Design review of the part built by this model. Coordinates are the model's own, in mm. A direction names the side the tool comes from. Coordinates: 2 decimals unless noted, no trailing zeros. Write item = value, one per line.
```python
from build123d import *

# Parameters (mm, degrees)
SKETCH_1_R          = 13
SKETCH_1_R_2        = 1.65
EXTRUDE_1_DEPTH     = 5
SKETCH_2_R          = 2
CUT_EXTRUDE_2_DEPTH = 5
CUT_EXTRUDE_START   = -5
CUT_EXTRUDE_3_DEPTH = 5
FILLET_1_R          = 2
FILLET_2_R          = 2
FILLET_3_R          = 2
CUT_EXTRUDE_5_DEPTH = 5
SKETCH_9_R          = 2
CUT_EXTRUDE_6_DEPTH = 10
SKETCH_10_R         = 2
CUT_EXTRUDE_7_DEPTH = 10
SKETCH_11_W         = 30
SKETCH_11_H         = 5
EXTRUDE_2_DEPTH     = 5
SKETCH_12_W         = 28.554441288
SKETCH_12_H         = 5
EXTRUDE_3_DEPTH     = 5


with BuildPart() as part:
    # 草图1 → 凸台-拉伸1 (new body)
    with BuildSketch(Plane.XY):
        with BuildLine():
            Line((0, 25), (450, 25))
            ThreePointArc((450, 25), (475, 0), (450, -25))
            Line((450, -25), (0, -25))
            ThreePointArc((0, -25), (-25, 0), (0, 25))
        make_face()
        Circle(SKETCH_1_R, mode=Mode.SUBTRACT)
        with Locations((17.5, 0)):
            Circle(SKETCH_1_R_2, mode=Mode.SUBTRACT)
        with Locations((0, -17.5)):
            Circle(SKETCH_1_R_2, mode=Mode.SUBTRACT)
        with Locations((-17.5, 0)):
            Circle(SKETCH_1_R_2, mode=Mode.SUBTRACT)
        with Locations((0, 17.5)):
            Circle(SKETCH_1_R_2, mode=Mode.SUBTRACT)
        with Locations((450, 0)):
            Circle(SKETCH_1_R, mode=Mode.SUBTRACT)
        with Locations((432.5, 0)):
            Circle(SKETCH_1_R_2, mode=Mode.SUBTRACT)
        with Locations((450, 17.5)):
            Circle(SKETCH_1_R_2, mode=Mode.SUBTRACT)
        with Locations((450, -17.5)):
            Circle(SKETCH_1_R_2, mode=Mode.SUBTRACT)
        with Locations((467.5, 0)):
            Circle(SKETCH_1_R_2, mode=Mode.SUBTRACT)
    extrude(amount=EXTRUDE_1_DEPTH)

    # 草图2 → 切除-拉伸2 (cut)
    with BuildSketch(Plane.XY.offset(5)):
        with Locations((290, 12.5)):
            Circle(SKETCH_2_R)
        with Locations((290, 0)):
            Circle(SKETCH_2_R)
        with Locations((290, -12.5)):
            Circle(SKETCH_2_R)
        with Locations((160, 12.5)):
            Circle(SKETCH_2_R)
        with Locations((160, 0)):
            Circle(SKETCH_2_R)
        with Locations((160, -12.5)):
            Circle(SKETCH_2_R)
    extrude(amount=-CUT_EXTRUDE_2_DEPTH, mode=Mode.SUBTRACT)

    # 草图4 → 切除-拉伸3 (cut)
    with BuildSketch(Plane.XY.offset(5).offset(CUT_EXTRUDE_START)):
        with BuildLine():
            Line((74.250402222, 0), (22.107690969, -17.5))
            ThreePointArc((22.107690969, -17.5), (20.333388811, -16.422958207), (20.470084231, -14.351851852))
            ThreePointArc((20.470084231, -14.351851852), (25, 0), (20.470084231, 14.351851852))
            ThreePointArc((20.470084231, 14.351851852), (20.333388811, 16.422958207), (22.107690969, 17.5))
            Line((22.107690969, 17.5), (74.250402222, 0))
        make_face()
        Polygon((82.107690969, -2.637042643), (126.393113474, -17.5), (37.822268465, -17.5), align=None)
        Polygon((37.822268465, 17.5), (126.393113474, 17.5), (82.107690969, 2.637042643), align=None)
        Polygon((142.107690969, 17.5), (142.107690969, -17.5), (89.964979717, 0), align=None)
    cut_extrude_3 = extrude(amount=CUT_EXTRUDE_3_DEPTH, mode=Mode.SUBTRACT)

    # 圆角1
    fillet_1_edges = [part.edges().sort_by_distance(p)[0] for p in [
        (142.107690969, 17.5, 2.5),
    ]]
    fillet(fillet_1_edges, radius=FILLET_1_R)

    # 圆角2
    fillet_2_edges = [part.edges().sort_by_distance(p)[0] for p in [
        (37.822268465, -17.5, 2.5),
        (82.107690969, -2.637042643, 2.5),
        (126.393113474, -17.5, 2.5),
        (89.964979717, 0, 2.5),
        (142.107690969, -17.5, 2.5),
        (126.393113474, 17.5, 2.5),
        (82.107690969, 2.637042643, 2.5),
        (37.822268465, 17.5, 2.5),
        (74.250402222, 0, 2.5),
    ]]
    fillet(fillet_2_edges, radius=FILLET_2_R)

    # 镜向1: 切除-拉伸3 across plane
    add(cut_extrude_3.mirror(Plane(origin=(225, 0, 0), x_dir=(0, 0, 1), z_dir=(1, 0, 0))), mode=Mode.SUBTRACT)

    # 圆角3
    fillet_3_edges = [part.edges().sort_by_distance(p)[0] for p in [
        (375.749597778, 0, 2.5),
        (367.892309031, -2.637042643, 2.5),
        (412.177731535, -17.5, 2.5),
        (323.606886526, -17.5, 2.5),
        (307.892309031, 17.5, 2.5),
        (360.035020283, 0, 2.5),
        (307.892309031, -17.5, 2.5),
        (367.892309031, 2.637042643, 2.5),
        (323.606886526, 17.5, 2.5),
        (412.177731535, 17.5, 2.5),
    ]]
    fillet(fillet_3_edges, radius=FILLET_3_R)

    # 草图8 → 切除-拉伸5 (cut)
    with BuildSketch(Plane.XY.offset(5)):
        with BuildLine():
            Line((198.641718603, 17.5), (251.358281397, 17.5))
            ThreePointArc((251.358281397, 17.5), (253.321552393, 15.881532429), (252.107332949, 13.645566994))
            Line((252.107332949, 13.645566994), (225.749051552, 2.998802443))
            ThreePointArc((225.749051552, 2.998802443), (225, 2.853235449), (224.250948448, 2.998802443))
            Line((224.250948448, 2.998802443), (197.892667051, 13.645566994))
            ThreePointArc((197.892667051, 13.645566994), (196.678447607, 15.881532429), (198.641718603, 17.5))
        make_face()
        with BuildLine():
            Line((175, 14.535156791), (175, -14.535156791))
            ThreePointArc((175, -14.535156791), (175.881541933, -16.193183193), (177.749051552, -16.389589796))
            Line((177.749051552, -16.389589796), (213.733857169, -1.854433006))
            ThreePointArc((213.733857169, -1.854433006), (214.984805617, 0), (213.733857169, 1.854433006))
            Line((213.733857169, 1.854433006), (177.749051552, 16.389589796))
            ThreePointArc((177.749051552, 16.389589796), (175.881541933, 16.193183193), (175, 14.535156791))
        make_face()
        with BuildLine():
            Line((198.641718603, -17.5), (251.358281397, -17.5))
            ThreePointArc((251.358281397, -17.5), (253.321552393, -15.881532429), (252.107332949, -13.645566994))
            Line((252.107332949, -13.645566994), (225.749051552, -2.998802443))
            ThreePointArc((225.749051552, -2.998802443), (225, -2.853235449), (224.250948448, -2.998802443))
            Line((224.250948448, -2.998802443), (197.892667051, -13.645566994))
            ThreePointArc((197.892667051, -13.645566994), (196.678447607, -15.881532429), (198.641718603, -17.5))
        make_face()
        with BuildLine():
            Line((275, 14.535156791), (275, -14.535156791))
            ThreePointArc((275, -14.535156791), (274.118458067, -16.193183193), (272.250948448, -16.389589796))
            Line((272.250948448, -16.389589796), (236.266142831, -1.854433006))
            ThreePointArc((236.266142831, -1.854433006), (235.015194383, 0), (236.266142831, 1.854433006))
            Line((236.266142831, 1.854433006), (272.250948448, 16.389589796))
            ThreePointArc((272.250948448, 16.389589796), (274.118458067, 16.193183193), (275, 14.535156791))
        make_face()
    extrude(amount=-CUT_EXTRUDE_5_DEPTH, mode=Mode.SUBTRACT)

    # 草图9 → 切除-拉伸6 (cut)
    with BuildSketch(Plane.XY.offset(5)):
        with Locations((38, 19)):
            Circle(SKETCH_9_R)
        with Locations((38, -19)):
            Circle(SKETCH_9_R)
    cut_extrude_6 = extrude(amount=-CUT_EXTRUDE_6_DEPTH, mode=Mode.SUBTRACT)

    # 镜向2: 切除-拉伸6 across plane
    add(cut_extrude_6.mirror(Plane(origin=(225, 0, 0), x_dir=(0, 0, 1), z_dir=(1, 0, 0))), mode=Mode.SUBTRACT)

    # 草图10 → 切除-拉伸7 (cut)
    with BuildSketch(Plane.XY.offset(5)):
        with Locations((126.148115476, 19)):
            Circle(SKETCH_10_R)
        with Locations((128.121960299, -19)):
            Circle(SKETCH_10_R)
    cut_extrude_7 = extrude(amount=-CUT_EXTRUDE_7_DEPTH, mode=Mode.SUBTRACT)

    # 镜向3: 切除-拉伸7 across plane
    add(cut_extrude_7.mirror(Plane(origin=(225, 0, 0), x_dir=(0, 0, 1), z_dir=(1, 0, 0))), mode=Mode.SUBTRACT)

    # 草图11 → 凸台-拉伸2 (add)
    with BuildSketch(Plane(origin=(0, 25, 0), x_dir=(1, 0, 0), z_dir=(0, 1, 0))):
        with Locations((225, -2.5)):
            Rectangle(SKETCH_11_W, SKETCH_11_H)
    extrude(amount=EXTRUDE_2_DEPTH)

    # 草图12 → 凸台-拉伸3 (add)
    with BuildSketch(Plane.XZ.offset(25)):
        with Locations((225, 2.5)):
            Rectangle(SKETCH_12_W, SKETCH_12_H)
    extrude(amount=EXTRUDE_3_DEPTH)


solid = part.part
```
(1) The part is to be moulded in two halves that separate along X. For faces 3 (the flat face through (98.989, 8.303, 2.465)), 4 (the cylindrical face through (-24.994, -0.55, 2.465)), 5 (the flat face through (228, 0, 5)), say which applies: released by +X, released by -X, zero draft, split by the parting line, or undercut.
Report:
face_3 = undercut
face_4 = released by -X
face_5 = zero draft
(2) Insertion check: pin 1 (1.5 mm diameter, centred on y = 28, z = 2.5, fed in from +X); pin 2 (4.5 mm diameter, centred on x = 290, y = 12.5, fed in from +Z); pin 3 (1 mm diameter, centred on x = 51, z = 3.5, fed in from +Y); pin 4 (2 mm diameter, centred on y = -14.5, z = 4, fed in from -X). Each pin has a flat end and moves straight along its axis. Give the tip position at first contact, or say it passes through.
Report:
pin_1 = 240
pin_2 = 5
pin_3 = 25
pin_4 = -21.04
(3) We need section A-A (z = 1.2). Give the number of separate pieces and of enclosed holes in the cut face, and give its area (3 significant figures).
Report:
separate_pieces = 1
enclosed_holes = 36
area = 14,900 mm²
(4) For faces 1 (the flat face through (404.971, 9.807, 2.465)), 2 (the flat face through (228, 0, 0)), list the 3-axis set-ups (+Z, -Z, +X, -X, +Y, -Y) from which the entire face can be reached by the end or side of a thin tool; tool diameter is ignored.
Report:
face_1 = +Z, -Z
face_2 = -Z, +X, -X, +Y, -Y
(5) For L1, parallel to Y at x = 0, z = 2.6; L2, parallel to Y at x = 38, z = 1.35; L3, parallel to Y at x = 81, z = 3.75, list the stretches that pass through material, from the lowest coordinate up.
Report:
L1 = -25 to -19.15, -15.85 to -13, 13 to 15.85, 19.15 to 25
L2 = -25 to -21, -17 to -12.17, 12.17 to 17, 21 to 25
L3 = -25 to -17.5, -3.01 to 3.01, 17.5 to 25
